Can you work these out from the model? Positions are in its coordinate system, mm. Give positions to 0.01 mm unless a question says otherwise; leave off trailing zeros. Order: outer loops, then holes, each group sorted by start corner. A loop starts at its lowest first (then second) coordinate and runs counter-clockwise, first axis right, second up.
```python
from build123d import *

# Parameters (mm, degrees)
SKETCH1_R           = 10
SKETCH1_R_2         = 1.972602619
BOSS_EXTRUDE2_DEPTH = 4
SKETCH5_W           = 5
SKETCH5_H           = 14
CUT_EXTRUDE3_DEPTH  = 5.0000001
SKETCH6_W           = 5
SKETCH6_H           = 14
CUT_EXTRUDE4_DEPTH  = 5.0000001
SKETCH19_R          = 2
CUT_EXTRUDE19_DEPTH = 5.0000001
SKETCH22_R          = 2
CUT_EXTRUDE22_DEPTH = 5.0000001
SKETCH23_R          = 2
CUT_EXTRUDE23_DEPTH = 5.0000001
SKETCH24_R          = 2
CUT_EXTRUDE24_DEPTH = 5.0000001
SKETCH25_W          = 5
SKETCH25_H          = 12
CUT_EXTRUDE25_DEPTH = 5.0000001
CUT_EXTRUDE26_DEPTH = 5.0000001
CUT_EXTRUDE29_DEPTH = 5.0000001
SKETCH20_R          = 2
CUT_EXTRUDE20_DEPTH = 5.0000001
SKETCH30_W          = 181.696441894
SKETCH30_H          = 131.456906608
CUT_EXTRUDE30_DEPTH = 4
SKETCH31_R          = 2
CUT_EXTRUDE31_DEPTH = 4
SKETCH32_W          = 167.461823271
SKETCH32_H          = 37.26795508
CUT_EXTRUDE32_DEPTH = 4
FILLET1_R           = 10
FILLET2_R           = 5
SKETCH33_W          = 2
SKETCH33_H          = 8
BOSS_EXTRUDE3_DEPTH = 4


with BuildPart() as part:
    # Sketch1 → Boss-Extrude2 (new body)
    with BuildSketch(Plane.XY):
        with BuildLine():
            Line((-49.4, 97.775402254), (-49.4, 48.775402254))
            Line((-49.4, 48.775402254), (-48.4, 48.775402254))
            Line((-48.4, 48.775402254), (-48.4, 35.775402254))
            Line((-48.4, 35.775402254), (-49.4, 35.775402254))
            Line((-49.4, 35.775402254), (-49.4, 21.775402254))
            Line((-49.4, 21.775402254), (-73.4, 21.775402254))
            Line((-73.4, 21.775402254), (-73.4, -12.924597746))
            Line((-73.4, -12.924597746), (-49.4, -12.924597746))
            Line((-49.4, -12.924597746), (-49.4, -26.924597746))
            Line((-49.4, -26.924597746), (-48.4, -26.924597746))
            Line((-48.4, -26.924597746), (-48.4, -39.924597746))
            Line((-48.4, -39.924597746), (-49.4, -39.924597746))
            Line((-49.4, -39.924597746), (-49.4, -88.924597746))
            Line((-49.4, -88.924597746), (-73.349457369, -88.924597746))
            add(Edge.make_bspline(
                [(-73.349457369, -88.924597746), (-70.502213021, -123.490651401), (3.447241601, -123.490651401), (77.396696223, -123.490651401), (74.549451875, -88.924597746)],
                knots=[3.190793702, 3.190793702, 3.190793702, 4.761590029, 4.761590029, 6.332386355, 6.332386355, 6.332386355], degree=2, weights=[1, 0.707106781, 1, 0.707106781, 1]))
            Line((74.549451875, -88.924597746), (50.599994505, -88.924597746))
            Line((50.599994505, -88.924597746), (50.599994505, -39.924597746))
            Line((50.599994505, -39.924597746), (49.599994505, -39.924597746))
            Line((49.599994505, -39.924597746), (49.599994505, -26.924597746))
            Line((49.599994505, -26.924597746), (50.599994505, -26.924597746))
            Line((50.599994505, -26.924597746), (50.599994505, -12.924597746))
            Line((50.599994505, -12.924597746), (74.599994505, -12.924597746))
            Line((74.599994505, -12.924597746), (74.599994505, 21.775402254))
            Line((74.599994505, 21.775402254), (50.669116659, 21.775402254))
            Line((50.669116659, 21.775402254), (50.669116659, 35.775402254))
            Line((50.669116659, 35.775402254), (49.669116659, 35.775402254))
            Line((49.669116659, 35.775402254), (49.669116659, 48.775402254))
            Line((49.669116659, 48.775402254), (50.669116659, 48.775402254))
            Line((50.669116659, 48.775402254), (50.669116659, 97.775402254))
            Line((50.669116659, 97.775402254), (74.669116659, 97.775402254))
            add(Edge.make_bspline(
                [(74.669116659, 97.775402254), (74.669116659, 132.775402254), (0.587265356, 132.775402254), (-73.494585946, 132.775402254), (-73.494585946, 97.775402254)],
                knots=[3.141592654, 3.141592654, 3.141592654, 4.71238898, 4.71238898, 6.283185307, 6.283185307, 6.283185307], degree=2, weights=[1, 0.707106781, 1, 0.707106781, 1]))
            Line((-73.494585946, 97.775402254), (-49.4, 97.775402254))
        make_face()
        with Locations((0, 72.732378713)):
            Circle(SKETCH1_R, mode=Mode.SUBTRACT)
        with Locations((0, -63.883577786)):
            Circle(SKETCH1_R, mode=Mode.SUBTRACT)
        with Locations((0, 4.424400463)):
            Circle(SKETCH1_R_2, mode=Mode.SUBTRACT)
    extrude(amount=BOSS_EXTRUDE2_DEPTH)

    # Sketch5 → Cut-Extrude3 (cut, through all)
    with BuildSketch(Plane(origin=(0, 0, 0), x_dir=(-1, 0, 0), z_dir=(0, 0, -1))):
        with Locations((46.9, 4.425402254)):
            Rectangle(SKETCH5_W, SKETCH5_H)
    extrude(amount=-CUT_EXTRUDE3_DEPTH, mode=Mode.SUBTRACT)

    # Sketch6 → Cut-Extrude4 (cut, through all)
    with BuildSketch(Plane(origin=(0, 0, 0), x_dir=(-1, 0, 0), z_dir=(0, 0, -1))):
        with Locations((-48.099994505, 4.425402254)):
            Rectangle(SKETCH6_W, SKETCH6_H)
    extrude(amount=-CUT_EXTRUDE4_DEPTH, mode=Mode.SUBTRACT)

    # Sketch19 → Cut-Extrude19 (cut, through all)
    with BuildSketch(Plane(origin=(0, 0, 0), x_dir=(-1, 0, 0), z_dir=(0, 0, -1))):
        with Locations((-56.599994505, 4.425402254)):
            Circle(SKETCH19_R)
    extrude(amount=-CUT_EXTRUDE19_DEPTH, mode=Mode.SUBTRACT)

    # Sketch22 → Cut-Extrude22 (cut, through all)
    with BuildSketch(Plane(origin=(0, 0, 0), x_dir=(-1, 0, 0), z_dir=(0, 0, -1))):
        with Locations((42.4, 81)):
            Circle(SKETCH22_R)
        with Locations((-43.669116659, 81)):
            Circle(SKETCH22_R)
    extrude(amount=-CUT_EXTRUDE22_DEPTH, mode=Mode.SUBTRACT)

    # Sketch23 → Cut-Extrude23 (cut, through all)
    with BuildSketch(Plane.XY.offset(4)):
        with Locations((43.599994505, -81)):
            Circle(SKETCH23_R)
        with Locations((-42.4, -81)):
            Circle(SKETCH23_R)
    extrude(amount=-CUT_EXTRUDE23_DEPTH, mode=Mode.SUBTRACT)

    # Sketch24 → Cut-Extrude24 (cut, through all)
    with BuildSketch(Plane.XY.offset(4)):
        with Locations((-50, -94.924597746)):
            Circle(SKETCH24_R)
        with Locations((50, -94.924597746)):
            Circle(SKETCH24_R)
        with Locations((-50, 103.775402254)):
            Circle(SKETCH24_R)
        with Locations((50, 103.775402254)):
            Circle(SKETCH24_R)
    extrude(amount=-CUT_EXTRUDE24_DEPTH, mode=Mode.SUBTRACT)

    # Sketch25 → Cut-Extrude25 (cut, through all)
    with BuildSketch(Plane(origin=(0, 0, 0), x_dir=(-1, 0, 0), z_dir=(0, 0, -1))):
        with Locations((-28.369116659, 42.275402254)):
            Rectangle(SKETCH25_W, SKETCH25_H)
        with Locations((27.1, 42.275402254)):
            Rectangle(SKETCH25_W, SKETCH25_H)
        with Locations((-28.299994505, -33.424597746)):
            Rectangle(SKETCH25_W, SKETCH25_H)
        with Locations((27.1, -33.424597746)):
            Rectangle(SKETCH25_W, SKETCH25_H)
    extrude(amount=-CUT_EXTRUDE25_DEPTH, mode=Mode.SUBTRACT)

    # Sketch26 → Cut-Extrude26 (cut, through all)
    with BuildSketch(Plane(origin=(0, 0, 0), x_dir=(-1, 0, 0), z_dir=(0, 0, -1))):
        Polygon((24.510151311, 52.075402254), (17.510151311, 52.075402254), (17.510151311, 59.075402254), (13.510151311, 59.075402254), (13.510151311, 66.075402254), (17.510151311, 66.075402254), (17.510151311, 73.075402254), (24.510151311, 73.075402254), (24.510151311, 66.075402254), (28.510151311, 66.075402254), (28.510151311, 59.075402254), (24.510151311, 59.075402254), align=None)
        Polygon((-29.999116659, 59.075402254), (-29.999116659, 66.075402254), (-25.999116659, 66.075402254), (-25.999116659, 73.075402254), (-18.999116659, 73.075402254), (-18.999116659, 66.075402254), (-14.999116659, 66.075402254), (-14.999116659, 59.075402254), (-18.999116659, 59.075402254), (-18.999116659, 52.075402254), (-25.999116659, 52.075402254), (-25.999116659, 59.075402254), align=None)
        Polygon((-19, -69), (-19, -62), (-15, -62), (-15, -55), (-19, -55), (-19, -48), (-26, -48), (-26, -55), (-30, -55), (-30, -62), (-26, -62), (-26, -69), align=None)
        Polygon((24.510151311, -48), (17.510151311, -48), (17.510151311, -55), (13.510151311, -55), (13.510151311, -62), (17.510151311, -62), (17.510151311, -69), (24.510151311, -69), (24.510151311, -62), (28.510151311, -62), (28.510151311, -55), (24.510151311, -55), align=None)
    extrude(amount=-CUT_EXTRUDE26_DEPTH, mode=Mode.SUBTRACT)

    # Sketch28 → Cut-Extrude29 (cut, through all)
    with BuildSketch(Plane(origin=(0, 0, 0), x_dir=(-1, 0, 0), z_dir=(0, 0, -1))):
        with BuildLine():
            Line((28.730883341, 86.928533544), (-30, 86.928533544))
            ThreePointArc((-30, 86.928533544), (-32, 88.928533544), (-30, 90.928533544))
            Line((-30, 90.928533544), (28.730883341, 90.928533544))
            ThreePointArc((28.730883341, 90.928533544), (30.730883341, 88.928533544), (28.730883341, 86.928533544))
        make_face()
    extrude(amount=-CUT_EXTRUDE29_DEPTH, mode=Mode.SUBTRACT)

    # Sketch20 → Cut-Extrude20 (cut, through all)
    with BuildSketch(Plane(origin=(0, 0, 0), x_dir=(-1, 0, 0), z_dir=(0, 0, -1))):
        with Locations((55.4, 4.425402254)):
            Circle(SKETCH20_R)
    extrude(amount=-CUT_EXTRUDE20_DEPTH, mode=Mode.SUBTRACT)

    # Sketch30 → Cut-Extrude30 (cut)
    with BuildSketch(Plane(origin=(0, 0, 0), x_dir=(-1, 0, 0), z_dir=(0, 0, -1))):
        with Locations((-2.534318945, -61.30305105)):
            Rectangle(SKETCH30_W, SKETCH30_H)
    extrude(amount=-CUT_EXTRUDE30_DEPTH, mode=Mode.SUBTRACT)

    # Sketch31 → Cut-Extrude31 (cut)
    with BuildSketch(Plane(origin=(0, 0, 0), x_dir=(-1, 0, 0), z_dir=(0, 0, -1))):
        with Locations((-18.412976441, 45.21289193)):
            Circle(SKETCH31_R)
        with Locations((-18.413659383, 8.47289193)):
            Circle(SKETCH31_R)
        with Locations((18.967023559, 45.21289193)):
            Circle(SKETCH31_R)
        with Locations((18.966340617, 8.47289193)):
            Circle(SKETCH31_R)
    extrude(amount=-CUT_EXTRUDE31_DEPTH, mode=Mode.SUBTRACT)

    # Sketch32 → Cut-Extrude32 (cut)
    with BuildSketch(Plane(origin=(0, 0, 0), x_dir=(-1, 0, 0), z_dir=(0, 0, -1))):
        with Locations((-4.661465148, 116.409379794)):
            Rectangle(SKETCH32_W, SKETCH32_H)
    extrude(amount=-CUT_EXTRUDE32_DEPTH, mode=Mode.SUBTRACT)

    # Fillet1
    fillet1_edges = [part.edges().sort_by_distance(p)[0] for p in [
        (-49.4, 97.775402254, 2),
        (50.669116659, 97.775402254, 2),
    ]]
    fillet(fillet1_edges, radius=FILLET1_R)

    # Fillet2
    fillet2_edges = [part.edges().sort_by_distance(p)[0] for p in [
        (74.599994505, 21.775402254, 2),
        (-73.4, 21.775402254, 2),
    ]]
    fillet(fillet2_edges, radius=FILLET2_R)

    # Sketch33 → Boss-Extrude3 (add)
    with BuildSketch(Plane.XY.offset(4)):
        with Locations((51.669116659, 52.775402254)):
            Rectangle(SKETCH33_W, SKETCH33_H)
        with Locations((51.669116659, 31.775402254)):
            Rectangle(SKETCH33_W, SKETCH33_H)
        with Locations((-50.4, 31.775402254)):
            Rectangle(SKETCH33_W, SKETCH33_H)
        with Locations((-50.4, 52.775402254)):
            Rectangle(SKETCH33_W, SKETCH33_H)
    extrude(amount=-BOSS_EXTRUDE3_DEPTH)

    # Mirror1: part across plane


with BuildPart() as part_1:
    add(part.part)
    add(part.part.mirror(Plane(origin=(0, 4.425402254, 0), x_dir=(0, 0, 1), z_dir=(0, -1, 0))))


solid = part_1.part
```
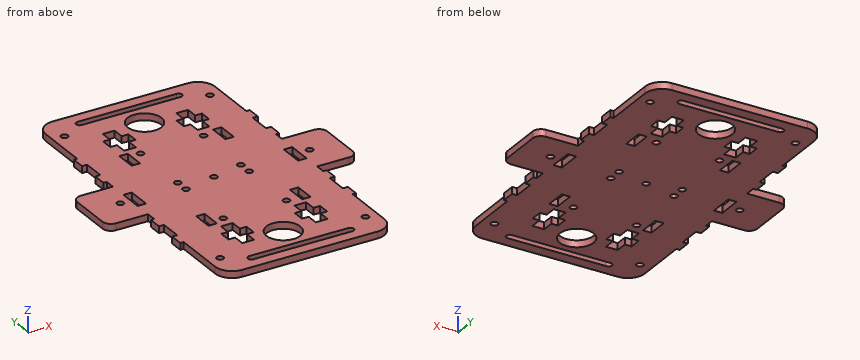
1) If I drill on line 1 (X direction, y = 62.5, z = 2.65); line 2 (X direction, y = -32, z = 1); line 3 (Y direction, x = 11, z = 2.25), over which ranges is the centre line in solid material (lowest first)?
2) I'm going to push flat-ended pins straight in: pin 1 Ø1 at (y, z) = (33, 3.5) entering from -X; pin 2 Ø1 at (x, z) = (-51, 1) entering from +Y; pin 3 Ø1 at (x, z) = (52, 1.5) entering from -Y. Where does each tip first touch, or does it pass through?
3) Suppose I cut it at C-C (x = -55.4). Please give me the cut outline in (y, z), and give its area (3 significant figures).
4) Suppose I cut it at D-D (z = 3.3). Give the number of separate pieces and of enclosed holes in the cut face, and give its area (3 significant figures).
5) Suppose I cut it at B-B (y = -32). Please give me the cut outline in (x, z), and give its area (3 significant figures).
6) Suppose I cut it at A-A (x = 0). Please give me the cut outline in (y, z).
Results:
1. line 1: x = -49.4 to -28.51, -13.51 to 15, 30 to 50.67
1. line 2: x = -48.4 to -29.6, -24.6 to 25.87, 30.87 to 49.67
1. line 3: y = -88.92 to -82.08, -78.08 to 86.93, 90.93 to 97.78
2. pin 1: stops at x = -51.4
2. pin 2: stops at y = 56.78
2. pin 3: stops at y = -47.92
3. outline: (-12.92, 0) - (2.43, 0) - (2.43, 4) - (-12.92, 4) - close; (6.43, 0) - (21.78, 0) - (21.78, 4) - (6.43, 4) - close
3. area: 123 mm2
4. separate pieces: 1
4. enclosed holes: 29
4. area: 17,800 mm2
5. outline: (-48.4, 0) - (-29.6, 0) - (-29.6, 4) - (-48.4, 4) - close; (-24.6, 0) - (25.87, 0) - (25.87, 4) - (-24.6, 4) - close; (30.87, 0) - (49.67, 0) - (49.67, 4) - (30.87, 4) - close
5. area: 352 mm2
6. outline: (-88.92, 0) - (-82.08, 0) - (-82.08, 4) - (-88.92, 4) - close; (-78.08, 0) - (-73.88, 0) - (-73.88, 4) - (-78.08, 4) - close; (-53.88, 0) - (2.45, 0) - (2.45, 4) - (-53.88, 4) - close; (6.4, 0) - (62.73, 0) - (62.73, 4) - (6.4, 4) - close; (82.73, 0) - (86.93, 0) - (86.93, 4) - (82.73, 4) - close; (90.93, 0) - (97.78, 0) - (97.78, 4) - (90.93, 4) - close
